Source: CAD feature listing. Evaluate the final solid. Frame: model axes, mm. A direction names the side the tool comes from. Round coordinates to 2 decimals unless told otherwise and drop trailing zeros. Loops run counter-clockwise (first coordinate to the right, second up) from the corner with the lowest first, then second, coordinate; pieces in that order, holes last. Notation, with made-up numbers: (67, 70.5) -> (113, 70.5) arc R18 cw to (113, 75.5) -> close; hole circle Ø8 at (-23.75, 9.25). An arc over 180 degrees is marked (long way). Put each result on its own line as item: value. Start each with the question number.
1. Cut plane C-C (x = -14). Return the cut outline in (y, z), then the cut area to 3 significant figures.
2. Cut plane B-B (x = 0.5). Return the cut outline in (y, z), then the cut area to 3 significant figures.
3. Material intervals for L1, parallel to Z at x = -10, y = 4.5; L2, parallel to Z at x = 20, y = 4.25; L3, parallel to Z at x = 13.5, y = 5.25, sorted ascending.
4. Draft query along X for faces 1 (the flat face through (23, 2, -7)), 2 (the flat face through (28, 4, -7)), 3 (the cylindrical face through (-13, 4, -14)), 4 (the flat face through (-32, 6, 0)). Return one class per face: pulls with the +X half, pulls with the -X half, needs draft (parallel to the pull), parting line crosses it, or undercut.
5. Set-up query: faces 5 (the cylindrical face through (13, 4, 14)), 6 (the flat face through (-12, 4, 0)), 7 (the flat face through (-30, 6.35, 0)), 8 (the flat face through (23, 6, 7)), 9 (the flat face through (23, 4, 9)). Return all of +Z, -Z, +X, -X, +Y, -Y with unobstructed straight access to the full face (end or side cutting, diameter ignored); none if empty.
6. Contact query for flat-ended pins moving along their axis: pin 1 (2 mm diameter, centred on x = 25, z = 7, fed in from -Y); pin 2 (1.5 mm diameter, centred on x = 21.5, z = 8, fed in from +Y); pin 3 (1.2 mm diameter, centred on x = 24, y = 3.5, fed in from +Z). Output: stop coordinate, or through.
```python
from build123d import *

# Parameters (mm, degrees)
BOSS_EXTRUDE1_DEPTH = 8
BOSS_EXTRUDE2_DEPTH = 4
SKETCH3_W           = 18
SKETCH3_H           = 2
CUT_EXTRUDE1_DEPTH  = 10
FILLET1_R           = 4
SKETCH4_W           = 9.5
SKETCH4_H           = 20
CUT_EXTRUDE2_DEPTH  = 4
SKETCH5_W           = 9.5
SKETCH5_H           = 20
CUT_EXTRUDE3_DEPTH  = 4


with BuildPart() as part:
    # Sketch1 → Boss-Extrude1 (new body)
    with BuildSketch(Plane(origin=(0, 0, 0), x_dir=(1, 0, 0), z_dir=(0, 1, 0))):
        with BuildLine():
            Line((-18, -10), (-18, -2))
            Line((-18, -2), (-28, -2))
            Line((-28, -2), (-28, 2))
            Line((-28, 2), (-18, 2))
            Line((-18, 2), (-18, 10))
            ThreePointArc((-18, 10), (-15.656854249, 15.656854249), (-10, 18))
            Line((-10, 18), (10, 18))
            ThreePointArc((10, 18), (15.656854249, 15.656854249), (18, 10))
            Line((18, 10), (18, 9))
            Line((18, 9), (28, 9))
            Line((28, 9), (28, 5))
            Line((28, 5), (18, 5))
            Line((18, 5), (18, -5))
            Line((18, -5), (28, -5))
            Line((28, -5), (28, -9))
            Line((28, -9), (18, -9))
            Line((18, -9), (18, -10))
            ThreePointArc((18, -10), (15.656854249, -15.656854249), (10, -18))
            Line((10, -18), (-10, -18))
            ThreePointArc((-10, -18), (-15.656854249, -15.656854249), (-18, -10))
        make_face()
        with BuildLine():
            Line((-10, -15), (10, -15))
            ThreePointArc((10, -15), (13.535533906, -13.535533906), (15, -10))
            ThreePointArc((15, -10), (12.658876757, -4.136567081), (6.923127464, -1.498028909))
            ThreePointArc((6.923127464, -1.498028909), (5.5, 0), (6.923127464, 1.498028909))
            ThreePointArc((6.923127464, 1.498028909), (12.658876757, 4.136567081), (15, 10))
            ThreePointArc((15, 10), (13.535533906, 13.535533906), (10, 15))
            Line((10, 15), (-10, 15))
            ThreePointArc((-10, 15), (-13.535533906, 13.535533906), (-15, 10))
            ThreePointArc((-15, 10), (-12.658876757, 4.136567081), (-6.923127464, 1.498028909))
            ThreePointArc((-6.923127464, 1.498028909), (-5.5, 0), (-6.923127464, -1.498028909))
            ThreePointArc((-6.923127464, -1.498028909), (-12.658876757, -4.136567081), (-15, -10))
            ThreePointArc((-15, -10), (-13.535533906, -13.535533906), (-10, -15))
        make_face(mode=Mode.SUBTRACT)
    extrude(amount=BOSS_EXTRUDE1_DEPTH)

    # Sketch2 → Boss-Extrude2 (add)
    with BuildSketch(Plane.ZY.offset(28)):
        Polygon((-1, 6.35), (2, 6.35), (2, 4.7), (-2, 4.7), (-2, 5.35), align=None)
    extrude(amount=BOSS_EXTRUDE2_DEPTH)

    # Sketch3 → Cut-Extrude1 (cut)
    with BuildSketch(Plane(origin=(28, 0, 0), x_dir=(0, 0, -1), z_dir=(1, 0, 0))):
        with Locations((0, 1)):
            Rectangle(SKETCH3_W, SKETCH3_H)
        with Locations((0, 7)):
            Rectangle(SKETCH3_W, SKETCH3_H)
    extrude(amount=-CUT_EXTRUDE1_DEPTH, mode=Mode.SUBTRACT)

    # Fillet1
    fillet1_edges = [part.edges().sort_by_distance(p)[0] for p in [
        (-28, 4.7, 0),
    ]]
    fillet(fillet1_edges, radius=FILLET1_R - 0.0001)  # a hair under: the kernel refuses the full size

    # Sketch4 → Cut-Extrude2 (cut)
    with BuildSketch(Plane.XZ):
        with Locations((10.25, 0)):
            Rectangle(SKETCH4_W, SKETCH4_H)
    extrude(amount=-CUT_EXTRUDE2_DEPTH, mode=Mode.SUBTRACT)

    # Sketch5 → Cut-Extrude3 (cut)
    with BuildSketch(Plane(origin=(0, 8, 0), x_dir=(1, 0, 0), z_dir=(0, 1, 0))):
        with Locations((-10.25, 0)):
            Rectangle(SKETCH5_W, SKETCH5_H)
    extrude(amount=-CUT_EXTRUDE3_DEPTH, mode=Mode.SUBTRACT)


solid = part.part
```
Solution:
1. outline: (0, -16.93) -> (8, -16.93) -> (8, -13) -> (0, -13) -> close; (0, -6) -> (4, -6) -> (4, 6) -> (0, 6) -> close; (0, 13) -> (8, 13) -> (8, 16.93) -> (0, 16.93) -> close
1. area: 111 mm^2
2. outline: (0, -18) -> (8, -18) -> (8, -15) -> (0, -15) -> close; (0, 15) -> (8, 15) -> (8, 18) -> (0, 18) -> close
2. area: 48.0 mm^2
3. L1: z = -18 to -15, 15 to 18
3. L2: z = -9 to -5, 5 to 9
3. L3: z = -17.19 to -13.57, -5.17 to 5.17, 13.57 to 17.19
4. face 1: needs draft
4. face 2: pulls with the +X half
4. face 3: undercut
4. face 4: pulls with the -X half
5. face 5: +Y, -Y
5. face 6: +Y
5. face 7: +Z, -Z, -X, +Y
5. face 8: +Z, -Z, +X, +Y
5. face 9: +Z, +X, +Y, -Y
6. pin 1: stops at y = 2
6. pin 2: stops at y = 6
6. pin 3: stops at z = 9
